Geometry: final body of the model. Coordinates: model frame, mm. Face numbers are marked on the shaded views. A direction names the side the tool comes from. Give positions to 0.01 mm unless a question says otherwise; leave off trailing zeros. Order: outer loops, then holes, each group sorted by start corner. A loop starts at its lowest first (then second) coordinate and runs counter-clockwise, first axis right, second up. Notation, with made-up numbers: (54, -18) -> (106, -18) arc R29 ccw to (106, 12) -> close; hole circle Ø7 at (13.25, 33). An arc over 180 degrees is marked (long way). Answer in a Markdown table with one row per item. Add a question column.
Q1. Contact query for flat-ended pins moving along their axis: P1, Ø4, axis at y = -105, z = -36, coming from the +X side; P2, Ø1, axis at x = -131, z = -43, coming from the -Y side; P3, Ø7, axis at x = -124, z = -37.5, coming from the +Y side. Output: stop coordinate, or through.
Q2. Cut plane A-A on z = -42.5. Return the cut outline in (x, y) (1 decimal), and give its area (3 significant figures).
Q3. Cut plane B-B on x = -126.5. Return the cut outline in (y, z).
Q4. Set-up query: the marked faces 1, 2 and 3. Return all of +Z, -Z, +X, -X, +Y, -Y with unobstructed straight access to the full face (end or side cutting, diameter ignored); none if empty.
Q5. Line query: line 1 along Y through (x, z) = (-127.5, -43). Output: solid intervals per line, ascending. Write a range as from..to.
Solid Edge part; units mm, degrees
sketch "Sketch1" plane through (-70.6437, 101.6, 0) normal (0, -1, 0) x (1, 0, 0)
  line L0 (-61.1187, -46.0375) -> (-46.8312, -46.0375)
  line L1 (-46.8312, -46.0375) -> (-46.8312, -26.9875)
  line L2 (-46.8312, -26.9875) -> (-61.1187, -26.9875)
  line L3 (-61.1187, -26.9875) -> (-61.1187, -46.0375)
  dimension "D1" = 46.8312
  dimension "D2" = 61.1187
extrude "Protrusion1" add sketch "Sketch1" along normal up to vertex (203.2 mm away)
sketch "Sketch2" plane through (-131.7625, 0, -34.1313) normal (-1, 0, 0) x (0, -1, 0)
  line L0 (-114.3, 7.1438) -> (114.3, 7.1438)
  line L1 (114.3, 7.1438) -> (114.3, -11.9063)
  line L2 (114.3, -11.9063) -> (-114.3, -11.9063)
  line L3 (-114.3, -11.9063) -> (-114.3, 7.1438)
extrude "Protrusion2" add sketch "Sketch2" along normal blind 4.7625
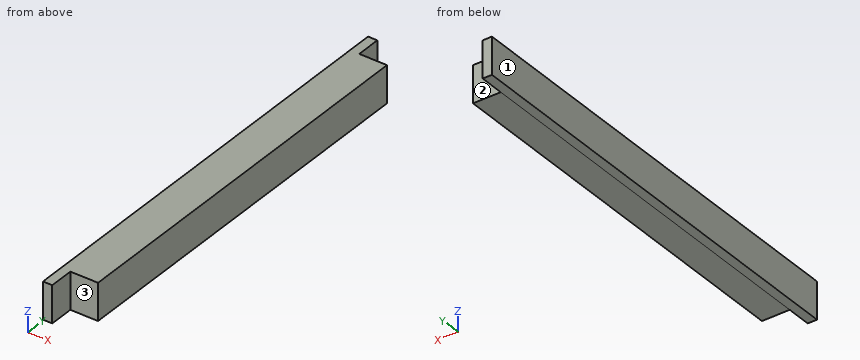
Completed:
| question | item | result |
|---|---|---|
| 1 | P1 | stops at x = -131.76 |
| 1 | P2 | stops at y = -101.6 |
| 1 | P3 | stops at y = 101.6 |
| 2 | outline | (-136.5, -114.3) -> (-131.8, -114.3) -> (-131.8, -101.6) -> (-117.5, -101.6) -> (-117.5, 101.6) -> (-131.8, 101.6) -> (-131.8, 114.3) -> (-136.5, 114.3) -> close |
| 2 | area | 3,990 mm² |
| 3 | outline | (-101.6, -46.04) -> (101.6, -46.04) -> (101.6, -26.99) -> (-101.6, -26.99) -> close |
| 4 | face 1 | +Z, -Z, -X, +Y, -Y |
| 4 | face 2 | +Z, -Z, +X, +Y |
| 4 | face 3 | +Z, -Z, +X, -Y |
| 5 | line 1 | y = -101.6..101.6 |
